Source: CAD feature listing. Evaluate the final solid. Frame: model axes, mm. A direction names the side the tool comes from. Give positions to 0.01 mm unless a question says otherwise; leave off trailing zeros. Write each loop counter-clockwise with the first axis right and the second up, starting at its lowest first coordinate (ties: lowest second). Pieces come first, ordered by that corner, then holes. Notation, with made-up numbers: M -20,14.25 L 36,14.25 A30 ccw 36,44.25 Z; hole C -39,-18.75 d9. An arc over 180 degrees is marked long. Use CSV: the item, a comma, the result in double quotes. Start each with the question number.
from build123d import *

# Parameters (mm, degrees)
SKETCH1_R           = 5
BOSS_EXTRUDE1_DEPTH = 5


with BuildPart() as part:
    # Sketch1 → Boss-Extrude1 (new body)
    with BuildSketch(Plane.XY):
        with BuildLine():
            Line((-202.232752641, -7.5), (-10.897247359, -7.5))
            ThreePointArc((-10.897247359, -7.5), (-7.543145393, -7.879808483), (-4.358898944, -9))
            ThreePointArc((-4.358898944, -9), (10, 0), (-4.358898944, 9))
            ThreePointArc((-4.358898944, 9), (-7.543145393, 7.879808483), (-10.897247359, 7.5))
            Line((-10.897247359, 7.5), (-202.232752641, 7.5))
            ThreePointArc((-202.232752641, 7.5), (-205.586854607, 7.879808483), (-208.771101056, 9))
            ThreePointArc((-208.771101056, 9), (-223.13, 0), (-208.771101056, -9))
            ThreePointArc((-208.771101056, -9), (-205.586854607, -7.879808483), (-202.232752641, -7.5))
        make_face()
        Circle(SKETCH1_R, mode=Mode.SUBTRACT)
        with BuildLine():
            Line((-213.13, 5), (-193.13, 5))
            ThreePointArc((-193.13, 5), (-188.13, 0), (-193.13, -5))
            Line((-193.13, -5), (-213.13, -5))
            ThreePointArc((-213.13, -5), (-218.13, 0), (-213.13, 5))
        make_face(mode=Mode.SUBTRACT)
    extrude(amount=BOSS_EXTRUDE1_DEPTH)


solid = part.part
1. Pull-direction query (X, two-part tool) for faces 5 (the flat face through (-108, 0, 5)), 6 (the cylindrical face through (-223.126, 0.283, 2.465)); classes: released by +X, released by -X, zero draft, split by the parting line, or undercut.
2. Section D-D on x = -148. Return loops of the section in (y, z).
3. Access query for faces 1 (the cylindrical face through (-188.13, 0.11, 2.46)), 2 (the flat face through (-105, 7.5, 2)), 3 (the flat face through (-108, 0, 0)), 4 (the cylindrical face through (-205.63, -7.89, 2.46)). Directions: +Z, -Z, +X, -X, +Y, -Y. A direction counts if a zero-diameter tool reaches every point of the face in a straight line with its end or side. Return the directions, or none.
4. Section B-B on z = 3.9. Return loops of the section in (x, y), then the cut area to 3 significant figures.
5. Line query: probe 1 along Y at (x, z) = (0, 1.9); probe 2 along Y at (x, z) = (-197, 1.5); probe 3 along X at (y, z) = (-0.75, 1.2). Output: solid intervals per line, ascending.
6. Section C-C on x = 0. Return loops of the section in (y, z).
7. First-contact query: pin 1 (3 mm diameter, centred on x = -35.5, z = 4.5, fed in from -Y); pin 2 (1.5 mm diameter, centred on x = -148, z = 1.5, fed in from +Y); pin 3 (2.5 mm diameter, centred on x = -203, z = 3, fed in from +Y); pin 4 (6 mm diameter, centred on x = 0, y = 0, fed in from -Z). Flat tips, straight axial feed; report the tip coordinate or a pass-through.
8. Section A-A on y = 0. Return loops of the section in (x, z), then the cut area to 3 significant figures.
Resolved:
1,face 5,"zero draft"
1,face 6,"undercut"
2,outline,"M -7.5,0 L 7.5,0 L 7.5,5 L -7.5,5 Z"
3,face 1,"+Z, -Z"
3,face 2,"+Z, -Z, +Y"
3,face 3,"-Z, +X, -X, +Y, -Y"
3,face 4,"+Z, -Z, -Y"
4,outline,"M -208.77,-9 A15 cw -202.23,-7.5 L -10.9,-7.5 A15 cw -4.36,-9 A10 ccw long -4.36,9 A15 cw -10.9,7.5 L -202.23,7.5 A15 cw -208.77,9 A10 ccw long Z; hole M -213.13,-5 L -193.13,-5 A5 ccw -193.13,5 L -213.13,5 A5 ccw Z; hole C 0,0 d10"
4,area,"3,200 mm2"
5,probe 1,"y = -10 to -5, 5 to 10"
5,probe 2,"y = -7.5 to -5, 5 to 7.5"
5,probe 3,"x = -223.1 to -218.07, -188.19 to -4.94, 4.94 to 9.97"
6,outline,"M -10,0 L -5,0 L -5,5 L -10,5 Z; M 5,0 L 10,0 L 10,5 L 5,5 Z"
7,pin 1,"stops at y = -7.5"
7,pin 2,"stops at y = 7.5"
7,pin 3,"stops at y = 7.64"
7,pin 4,"passes through"
8,outline,"M -223.13,0 L -218.13,0 L -218.13,5 L -223.13,5 Z; M -188.13,0 L -5,0 L -5,5 L -188.13,5 Z; M 5,0 L 10,0 L 10,5 L 5,5 Z"
8,area,"966 mm2"
